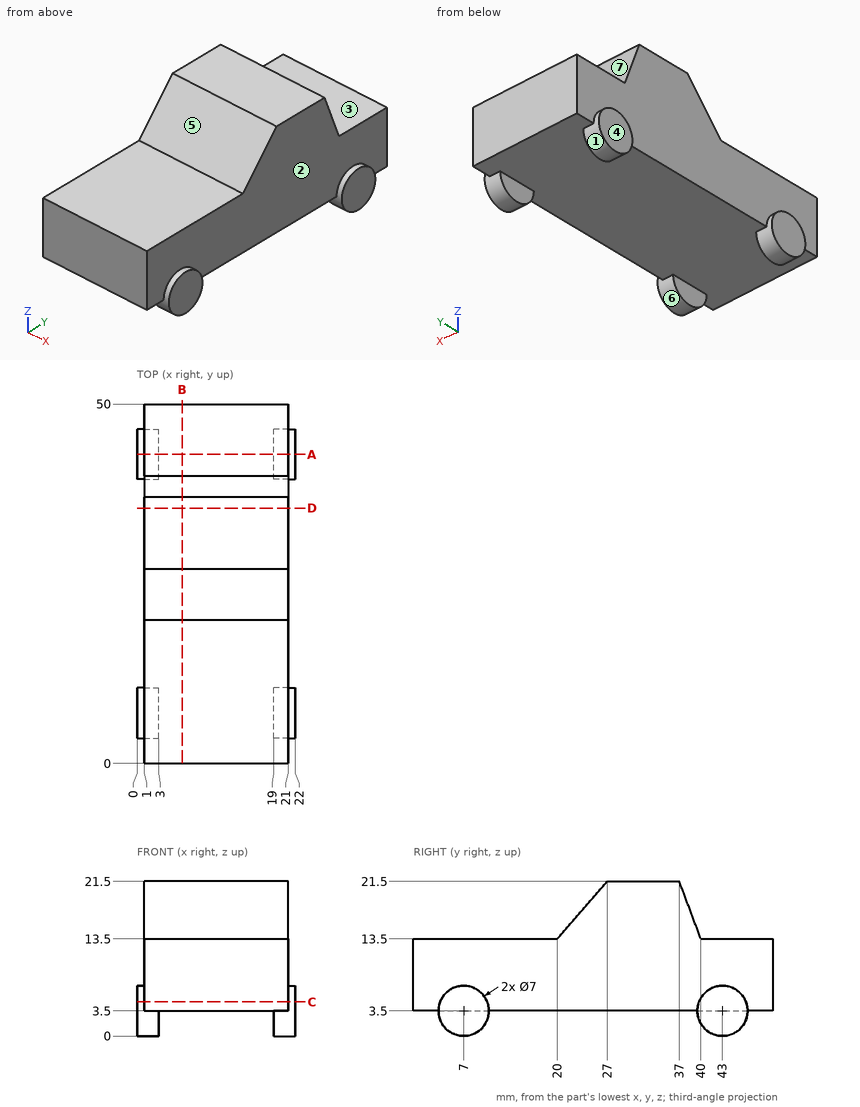
The drawing under review shows one solid part. Ordinate dimensions are in mm from its lowest x, y, z. A direction names the side the tool comes from. Round coordinates to 2 decimals unless told otherwise and drop trailing zeros. Write each loop counter-clockwise with the first axis right and the second up, starting at its lowest first coordinate (ties: lowest second). Pieces come first, ordered by that corner, then holes. Notation, with made-up numbers: (-35.75, 75.5) - (1.25, 75.5) arc R25 cw to (1.25, 89.5) - close; hole circle Ø9 at (-2.5, 38.25). An arc over 180 degrees is marked (long way). Use one line per item in the form item = value.
Q1. Draft analysis for pull direction Y (two halves, no side actions). For the marked faces 4, 5, 6 and 7, state which applies: +Y half, -Y half, draft (parallel to the pull), parting line (faces both ways), or undercut.
Answer key:
face_4 = draft
face_5 = -Y half
face_6 = undercut
face_7 = +Y half
Q2. Consider section D-D (y = 35.5). State the section outline as (x, z) points.
Answer key:
outline = (1, 3.5) - (21, 3.5) - (21, 21.5) - (1, 21.5) - close
Q3. For line 1 (Z direction, x = 4.25, y = 43); line 2 (Z direction, x = 2, y = 36); line 3 (X direction, y = 23.5, z = 6.5), list the stretches that pass through material, from the lowest coordinate up. Write a range as [from, to].
Answer key:
line_1 = [3.5, 13.5]
line_2 = [3.5, 21.5]
line_3 = [1, 21]
Q4. Consider section A-A (y = 43). State the section outline as (x, z) points, and give its area (3 significant figures).
Answer key:
outline = (0, 0) - (3, 0) - (3, 3.5) - (19, 3.5) - (19, 0) - (22, 0) - (22, 7) - (21, 7) - (21, 13.5) - (1, 13.5) - (1, 7) - (0, 7) - close
area = 228 mm2
Q5. Insertion check: pin 1 Ø1 at (y, z) = (44, 8.5) entering from +X; pin 2 Ø8 at (x, y) = (14, 46.5) entering from +Z. Each pin has a flat end and moves straight along its axis. Give the tip position at first contact, or say it passes through.
Answer key:
pin_1 = 21
pin_2 = 13.5
Q6. Consider section C-C (z = 4.75). State the section outline as (x, y) points.
Answer key:
outline = (0, 3.73) - (1, 3.73) - (1, 0) - (21, 0) - (21, 3.73) - (22, 3.73) - (22, 10.27) - (21, 10.27) - (21, 39.73) - (22, 39.73) - (22, 46.27) - (21, 46.27) - (21, 50) - (1, 50) - (1, 46.27) - (0, 46.27) - (0, 39.73) - (1, 39.73) - (1, 10.27) - (0, 10.27) - close
Q7. Tool access review of the marked faces 1, 2 and 3: name each direction out of +Z, -Z, +X, -X, +Y, -Y from which nothing blocks a thin tool from reaching the whole face with its end or side.
Answer key:
face_1 = -X
face_2 = +Z, +X
face_3 = +Z, +X, -X, +Y
Q8. Consider section B-B (x = 6.25). State the section outline as (y, z) points.
Answer key:
outline = (0, 3.5) - (50, 3.5) - (50, 13.5) - (40, 13.5) - (37, 21.5) - (27, 21.5) - (20, 13.5) - (0, 13.5) - close
